from build123d import *

# Parameters (mm, degrees)
SKETCH1_R           = 1.5
BOSS_EXTRUDE1_DEPTH = 6.4
BOSS_EXTRUDE2_DEPTH = 2.38
SKETCH3_R           = 2.185
BOSS_EXTRUDE3_DEPTH = 3.97
BOSS_EXTRUDE4_DEPTH = 8.73
FILLET1_R           = 0.7


with BuildPart() as part:
    # Sketch1 → Boss-Extrude1 (new body)
    with BuildSketch(Plane.XY):
        Circle(SKETCH1_R)
    extrude(amount=BOSS_EXTRUDE1_DEPTH)

    # Sketch2 → Boss-Extrude2 (add)
    with BuildSketch(Plane.XY.offset(6.4)):
        Polygon((1.374093641, -2.38), (2.748187281, 0), (1.374093641, 2.38), (-1.374093641, 2.38), (-2.748187281, 0), (-1.374093641, -2.38), align=None)
    extrude(amount=BOSS_EXTRUDE2_DEPTH)

    # Sketch3 → Boss-Extrude3 (add)
    with BuildSketch(Plane.XY.offset(8.78)):
        Circle(SKETCH3_R)
    extrude(amount=BOSS_EXTRUDE3_DEPTH)

    # Sketch4 → Boss-Extrude4 (add)
    with BuildSketch(Plane.XY.offset(12.75)):
        with BuildLine():
            Line((-0.9, 0.8), (0.9, 0.8))
            ThreePointArc((0.9, 0.8), (1.7, 0), (0.9, -0.8))
            Line((0.9, -0.8), (-0.9, -0.8))
            ThreePointArc((-0.9, -0.8), (-1.7, 0), (-0.9, 0.8))
        make_face()
    extrude(amount=BOSS_EXTRUDE4_DEPTH)

    # Fillet1
    fillet1_edges = [part.edges().sort_by_distance(p)[0] for p in [
        (-1.7, 0, 21.48),
        (0, -0.8, 21.48),
        (1.7, 0, 21.48),
        (0, 0.8, 21.48),
    ]]
    fillet(fillet1_edges, radius=FILLET1_R)


solid = part.part
The listing builds one solid part. Answer for the finished solid, in the listing's coordinates (mm). A direction names the side the tool comes from. Coordinates: 2 decimals unless noted, no trailing zeros. Order: outer loops, then holes, each group sorted by start corner. A loop starts at its lowest first (then second) coordinate and runs counter-clockwise, first axis right, second up. Notation, with made-up numbers: (8.5, 78) -> (29.5, 78) arc R28 ccw to (29.5, 111) -> close; hole circle Ø1 at (-24.5, 20). An arc over 180 degrees is marked (long way). Answer in a Markdown table with one row per item. Add a question column.
Item 1: Find section A-A (x = 0). Write down the section's boundary in (y, z) (3 decimals), then the cut area to 3 significant figures.
Item 2: Find the intervals of material crossed by L1, parallel to Y at x = 0.85, z = 16; L2, parallel to Z at x = 0.65, y = 1.7; L3, parallel to Z at x = -2.05, y = 1, in increasing order. Write a range as from..to.
Item 3: Find section B-B (y = 1.7). Write down the section's boundary in (x, z), then the cut area to 3 significant figures.
Item 4: Each of these flat-tipped pins is pushed along its axis until it touches: P1, Ø1, axis at x = 0, z = 11.5, coming from the -Y side (3 decimals); P2, Ø2, axis at x = 0, z = 17, coming from the +Y side; P3, Ø1.4, axis at x = 0.5, z = 18.5, coming from the -Y side. Where does it stop, or does it pass through?
Item 5: Find section C-C (z = 8). Write down the section's boundary in (x, y).
Item 6: Which of the six approach directions +Z, -Z, +X, -X, +Y, -Y give full straight-line access (tool end or side, diameter ignored) to faces 1 (the face through (0, -0.8, 17)), 2 (the face through (-1.7, 0, 16.7)), 3 (the face through (2.084, 0.656, 10.737)), 4 (the face through (-1.5, 0.07, 3.16))?
Item 7: Find section D-D (z = 12.5). Write down the section's boundary in (x, y) (3 decimals), then the cut area to 3 significant figures.
Result set:
| question | item | result |
|---|---|---|
| 1 | outline | (-2.38, 6.4) -> (-1.5, 6.4) -> (-1.5, 0) -> (1.5, 0) -> (1.5, 6.4) -> (2.38, 6.4) -> (2.38, 8.78) -> (2.185, 8.78) -> (2.185, 12.75) -> (0.8, 12.75) -> (0.8, 20.78) arc R0.7 ccw to (0.1, 21.48) -> (-0.1, 21.48) arc R0.7 ccw to (-0.8, 20.78) -> (-0.8, 12.75) -> (-2.185, 12.75) -> (-2.185, 8.78) -> (-2.38, 8.78) -> close |
| 1 | area | 61.6 mm² |
| 2 | L1 | y = -0.8..0.8 |
| 2 | L2 | z = 6.4..12.75 |
| 2 | L3 | z = 6.4..8.78 |
| 3 | outline | (-1.77, 6.4) -> (1.77, 6.4) -> (1.77, 8.78) -> (1.37, 8.78) -> (1.37, 12.75) -> (-1.37, 12.75) -> (-1.37, 8.78) -> (-1.77, 8.78) -> close |
| 3 | area | 19.3 mm² |
| 4 | P1 | stops at y = -2.185 |
| 4 | P2 | stops at y = 0.8 |
| 4 | P3 | stops at y = -0.8 |
| 5 | outline | (-2.75, 0) -> (-1.37, -2.38) -> (1.37, -2.38) -> (2.75, 0) -> (1.37, 2.38) -> (-1.37, 2.38) -> close |
| 6 | face 1 | +Z, +X, -X, -Y |
| 6 | face 2 | +Z, -X |
| 6 | face 3 | +Z |
| 6 | face 4 | -Z |
| 7 | outline | circle Ø4.37 at (0, 0) |
| 7 | area | 15.0 mm² |
